Input: part model. Units: mm. Frame: model coordinates. A direction names the side the tool comes from. Round coordinates to 2 decimals unless told otherwise and drop trailing zeros. Loops run counter-clockwise (first coordinate to the right, second up) from the corner with the lowest first, then second, coordinate; pieces in that order, holes last.
1) Section A-A, the plane x = 59.25. Return loops of the section in (y, z).
2) Section D-D, the plane z = 5. Return loops of the section in (x, y).
3) Draft query along Z for faces 1 (the face through (54.754, 47.098, -13.343)), 2 (the face through (62.26, 12.054, -8.64)), 3 (the face through (54.754, -47.098, 5.243)). Return one class per face: pulls with the +Z half, pulls with the -Z half, needs draft (parallel to the pull), parting line crosses it, or undercut.
4) First-contact query: pin 1 (1.6 mm diameter, centred on y = -41.41, z = -10.51, fed in from +X); pin 2 (12 mm diameter, centred on y = 9.5, z = -5.5, fed in from -X); pin 3 (11 mm diameter, centred on y = -23.53, z = -3, fed in from +X). Flat tips, straight axial feed; report the tip coordinate or a pass-through.
5) Access query for faces 4 (the face through (58, 46.2, -4)), 5 (the face through (58.8, -47.29, -13.53)). Directions: +Z, -Z, +X, -X, +Y, -Y. A direction counts if a zero-diameter tool reaches every point of the face in a straight line with its end or side. Return the directions, or none.
6) Section B-B, the plane y = -21.5. Return loops of the section in (x, z), and give its area (3 significant figures).
7) Ray query, line 1 along Y through (x, z) = (59, -4.5); line 2 along Z through (x, y) = (60, -39); line 3 along Y through (x, z) = (61.75, 1.75) (3 decimals). Return the intervals inside material, ascending.
8) Section C-C, the plane y = 38. Return loops of the section in (x, z).
from build123d import *

# Parameters (mm, degrees)
SKETCH014_R             = 2.175
SKETCH014_R_2           = 1
SKETCH014_R_3           = 3.375
SKETCH014_R_4           = 0.9
PAD012_DEPTH            = 1.5
PAD013_DEPTH            = 1.5
PAD013_DEPTH_BACK       = 7
CHAMFER_SIZE            = 0.9
CHAMFER001_SIZE         = 0.5
CHAMFER002_SIZE         = 0.5
CHAMFER003_SIZE         = 0.4
BODY003_PLACEMENT_ANGLE = 180


with BuildPart() as part:
    # Sketch014 → Pad012 (new body)
    with BuildSketch(Plane.YZ.offset(60)):
        Polygon((-44.238463, 6.7), (44.238463, 6.7), (46.2, 1.310722), (46.2, -9.910722), (44.238463, -15.3), (-44.238463, -15.3), (-46.2, -9.910722), (-46.2, 1.310722), align=None)
        with Locations((-26.058118, -6.71)):
            Circle(SKETCH014_R, mode=Mode.SUBTRACT)
        with Locations((-19.558118, -1.5)):
            Circle(SKETCH014_R_2, mode=Mode.SUBTRACT)
        with Locations((-13.058118, -6.71)):
            Circle(SKETCH014_R, mode=Mode.SUBTRACT)
        with Locations((-6.908118, -1.5)):
            Circle(SKETCH014_R_2, mode=Mode.SUBTRACT)
        with Locations((-2.338118, -1.5)):
            Circle(SKETCH014_R_2, mode=Mode.SUBTRACT)
        with Locations((2.231882, -1.5)):
            Circle(SKETCH014_R_2, mode=Mode.SUBTRACT)
        with Locations((6.801882, -1.5)):
            Circle(SKETCH014_R_2, mode=Mode.SUBTRACT)
        with Locations((11.371882, -1.5)):
            Circle(SKETCH014_R_2, mode=Mode.SUBTRACT)
        with Locations((23.531882, -3)):
            Circle(SKETCH014_R_3, mode=Mode.SUBTRACT)
        with Locations((-41.409188, 1.909188)):
            Circle(SKETCH014_R_4, mode=Mode.SUBTRACT)
        with Locations((41.409188, 1.909188)):
            Circle(SKETCH014_R_4, mode=Mode.SUBTRACT)
        with Locations((41.409188, -10.509188)):
            Circle(SKETCH014_R_4, mode=Mode.SUBTRACT)
        with Locations((-41.409188, -10.509188)):
            Circle(SKETCH014_R_4, mode=Mode.SUBTRACT)
    extrude(amount=PAD012_DEPTH)

    # Sketch015 (on Face23 of Pad012) → Pad013 (join, two sides)
    with BuildSketch(Plane.YZ.offset(61.5)) as pad013_sk:
        Polygon((-45.91953, 9.2), (-48.7, 1.560722), (-48.7, -9.660722), (-45.91953, -17.3), (45.91953, -17.3), (48.7, -9.660722), (48.7, 1.560722), (45.91953, 9.2), align=None)
        Polygon((-44.238463, 6.7), (44.238463, 6.7), (46.2, 1.310722), (46.2, -9.910722), (44.238463, -15.3), (-44.238463, -15.3), (-46.2, -9.910722), (-46.2, 1.310722), align=None, mode=Mode.SUBTRACT)
    extrude(amount=-PAD013_DEPTH)
    extrude(pad013_sk.sketch, amount=PAD013_DEPTH_BACK)

    # Chamfer
    chamfer_edges = [part.edges().sort_by_distance(p)[0] for p in [
        (60, -42.309188, -10.509188),
        (60, -42.309188, 1.909188),
        (60, 40.509188, 1.909188),
        (60, 40.509188, -10.509188),
    ]]
    chamfer(chamfer_edges, length=CHAMFER_SIZE)

    # Chamfer001
    chamfer001_edges = [part.edges().sort_by_distance(p)[0] for p in [
        (68.5, 0, 6.7),
        (68.5, -45.219232, 4.005361),
        (68.5, -46.2, -4.3),
        (68.5, -45.219232, -12.605361),
        (68.5, 0, -15.3),
        (68.5, 45.219232, -12.605361),
        (68.5, 46.2, -4.3),
        (68.5, 45.219232, 4.005361),
    ]]
    chamfer(chamfer001_edges, length=CHAMFER001_SIZE)

    # Chamfer002
    chamfer002_edges = [part.edges().sort_by_distance(p)[0] for p in [
        (68.5, 0, 9.2),
        (68.5, -47.309765, 5.380361),
        (68.5, -48.7, -4.05),
        (68.5, -47.309765, -13.480361),
        (68.5, 0, -17.3),
        (68.5, 47.309765, -13.480361),
        (68.5, 48.7, -4.05),
        (68.5, 47.309765, 5.380361),
        (60, 47.309765, 5.380361),
        (60, 48.7, -4.05),
        (60, 47.309765, -13.480361),
        (60, 0, -17.3),
        (60, 0, 9.2),
        (60, -47.309765, 5.380361),
        (60, -48.7, -4.05),
        (60, -47.309765, -13.480361),
    ]]
    chamfer(chamfer002_edges, length=CHAMFER002_SIZE)

    # Chamfer003
    chamfer003_edges = [part.edges().sort_by_distance(p)[0] for p in [
        (60, -7.908118, -1.5),
        (60, -3.338118, -1.5),
        (60, 1.231882, -1.5),
        (60, 5.801882, -1.5),
        (60, 10.371882, -1.5),
    ]]
    chamfer(chamfer003_edges, length=CHAMFER003_SIZE)


with BuildPart() as part_1:
    # Body003 placement: moved
    add(part.part.moved(Location((123, 0, 0))).rotate(Axis((123, 0, 0), (0, 0, 1)), BODY003_PLACEMENT_ANGLE))


solid = part_1.part
Final values:
1. outline: (-48.7, -9.66) - (-45.92, -17.3) - (45.92, -17.3) - (48.7, -9.66) - (48.7, 1.56) - (45.92, 9.2) - (-45.92, 9.2) - (-48.7, 1.56) - close; hole (-46.2, -9.91) - (-44.24, -15.3) - (44.24, -15.3) - (46.2, -9.91) - (46.2, 1.31) - (44.24, 6.7) - (-44.24, 6.7) - (-46.2, 1.31) - close
2. outline: (54.5, -46.92) - (55, -47.45) - (62.5, -47.45) - (63, -46.92) - (63, 46.92) - (62.5, 47.45) - (55, 47.45) - (54.5, 46.92) - (54.5, 45.39) - (55, 44.86) - (61.5, 44.86) - (61.5, -44.86) - (55, -44.86) - (54.5, -45.39) - close
3. face 1: pulls with the -Z half
3. face 2: undercut
3. face 3: pulls with the +Z half
4. pin 1: passes through
4. pin 2: stops at x = 61.5
4. pin 3: stops at x = 63
5. face 4: -X
5. face 5: -Z, +X, -X, -Y
6. outline: (54.5, -16.8) - (55, -17.3) - (62.5, -17.3) - (63, -16.8) - (63, -5.69) - (61.5, -5.69) - (61.5, -15.3) - (55, -15.3) - (54.5, -15.8) - close; (54.5, 7.2) - (55, 6.7) - (61.5, 6.7) - (61.5, -0.31) - (63, -0.31) - (63, 8.7) - (62.5, 9.2) - (55, 9.2) - (54.5, 8.7) - close
6. area: 62.4 mm2
7. line 1: y = -48.7 to -46.2, 46.2 to 48.7
7. line 2: z = -17.3 to -15.3, 6.7 to 9.2
7. line 3: y = -48.631 to -42.295, -40.523 to 40.523, 42.295 to 48.631
8. outline: (54.5, -16.8) - (55, -17.3) - (62.5, -17.3) - (63, -16.8) - (63, 8.7) - (62.5, 9.2) - (55, 9.2) - (54.5, 8.7) - (54.5, 7.2) - (55, 6.7) - (61.5, 6.7) - (61.5, -15.3) - (55, -15.3) - (54.5, -15.8) - close
